Autodesk Inventor part; units mm, degrees
ref_plane "IDS_WORKPLANE{1}" through (-1.5513, 0, 0) normal (1, 0, 0) x (0, 0, -1)
ref_plane "Work Plane2" through (8.25, 0, 0) normal (0, 0, -1) x (1, 0, 0)
ref_plane "YZ Plane" through (0, 0, 0) normal (1, 0, 0) x (0, 1, 0)
sketch "Sketch1" plane through (0, 0, 0) normal (0, 0, 1) x (1, 0, 0)
  line L0 (-1.5513, 0) -> (5, 0)
  line L1 (5, 0) -> (5, 1.15)
  line L2 (5, 1.15) -> (1, 1.15)
  line L3 (1, 1.15) -> (0.7546, 1.0272)
  line L4 (0.7546, 1.0272) -> (0, 1.0272)
  line L5 (0, 1.0272) -> (0, 2)
  line L6 (-5.4046, 0) -> (21.3851, 0)
  line L7 (0, -0.4002) -> (0, 2.4013)
  line L8 (0, 2) -> (-1.4463, 1.9997)
  arc A0 (-1.4463, 1.9997) -> (-1.5513, 0) centre (17.558, 0) ccw
  dimension "d0" = 5
  dimension "d1" = 4
  dimension "d2" = 0.2454
  dimension "d3" = 1.5513
  dimension "d4" = 2.3
  dimension "d5" = 2.0545
  dimension "d9" = 4
  dimension "d10" = 0.01
  dimension "d15" = 19.1093
revolve "Body" add sketch "Sketch1" angle 360 about axis through (-1.5513, 0, 0) along (1, 0, 0)
fillet "Fillet1" radius 1.3 1 edges at (-1.4463, -1.9997, 0)
ref_plane "IDS_WORKPLANE{1}" through (-1.5513, 0, 0) normal (1, 0, 0) x (0, 0, -1)
sketch "Sketch2" plane through (-1.5513, 0, 0) normal (1, 0, 0) x (0, 0, -1)
  line L0 (0, -2.8) -> (0, 2.8)
  line L1 (2.8, 0) -> (-2.8, 0)
  line L2 (-2, 0.3) -> (2, 0.3)
  line L3 (2, 0.3) -> (2, -0.3)
  line L4 (2, -0.3) -> (-2, -0.3)
  line L5 (-2, -0.3) -> (-2, 0.3)
  line L6 (0, 0.3) -> (0, -0.3) construction
  line L7 (-2, 0) -> (2, 0) construction
  circle A0 centre (0, 0) radius 2
  dimension "d17" = 0.6
extrude "Slot" cut sketch "Sketch2" along normal blind 0.9 contours L4 A0 L1 L0 | L0 L1 A0 L4 | L4 L5 A0 | A0 L3 L4 | L1 A0 L2 L0 | L0 L2 A0 L1 | L5 L2 A0 | A0 L2 L3
thread "Thread"
chamfer "Chamfer1" distance 0.2454 distance2 0.2455 1 edges at (5, -1.15, 0) measured on face at (5, 0.3197, -0.0157)
ref_plane "Work Plane2" through (8.25, 0, 0) normal (0, 0, -1) x (1, 0, 0)
equation "\"d0\" = NLG"
equation "\"d1\" = GEL"
equation "\"d2\" = GAL"
equation "\"d3\" = KOH"
equation "\"d4\" = GD"
equation "\"d5\" = BDM"
equation "\"d9\" = KOD"
equation "\"d10\" = KEWI"
equation "\"d17\" = SBR"
equation "\"d18\" = STI"
equation "\"d20\" = RR"
equation "\"d11\" = GEL"
equation "\"d13\" = -0.5 * SPD + 0.5 * GD"
equation "\"GD\" = NND"
equation "\"NLG\" = 5"
equation "\"GEL\" = 4"
equation "\"KOD\" = 4"
equation "\"KOH\" = 1.55125"
equation "\"GAL\" = 0.61345 * PTC"
equation "\"SPD\" = NND - 1.2269 * PTC"
equation "\"BDM\" = 2.0545"
equation "\"GUL\" = 0.61345 * PTC"
equation "\"RR\" = 1.3"
equation "\"SBR\" = 0.6"
equation "\"STI\" = 0.9"
equation "\"KEWI\" = 0.01deg"
equation "\"KR\" = 2.4"
equation "\"d16\" = -KOH"
equation "\"PTC\" = 0.4"
equation "\"THREADDIA\" = 2.3"
equation "\"TOA\" = 30deg"
equation "\"NND\" = 2.3"
equation "\"ORI\" = 1.3"
equation "\"GD1\" = THREADDIA - 1.2269 * PTC"
properties part number "CNS 9671 - M2.3 x 5" material "Steel, Mild"
Check sheet for the modelled part. Datum: model origin and axes. Units: mm. A direction names the side the tool comes from. Round coordinates to 2 decimals unless told otherwise and drop trailing zeros. Write each loop counter-clockwise with the first axis right and the second up, starting at its lowest first coordinate (ties: lowest second). Pieces come first, ordered by that corner, then holes. Notation, with made-up numbers: M 79,-34 L 124,-34 A19 ccw 124,-11 Z; hole C -16,-29 d10. An arc over 180 degrees is marked long. Write item = value, one per line. Start each with the question number.
1. Gauge pin test, flat ends, axial feed: pin 1 (1.5 mm diameter, centred on x = 1.5, y = -0.5, fed in from +Z); pin 2 (0.7 mm diameter, centred on x = -1.5, z = 1, fed in from +Y); pin 3 (1 mm diameter, centred on x = -1, z = 0.5, fed in from -Y). Record the tip position at first contact, or that the pin passes through.
2. Section check A-A, the plane x = 4.5. Record the cut outline in (y, z).
3. Scan lines: line 1 (Y direction, x = 0.5, z = 0.05); line 2 (X direction, y = -0.4, z = 0.6); line 3 (Z direction, x = 4.5, y = -0.1). Record each from-to range of solid material in increasing order. Write a range as [from, to].
4. Tool access check on faces 1 (the cylindrical face through (2.85, -0.91, 0.7)), 2 (the flat face through (5, 0, 0)), 3 (the flat face through (-1, 0.3, 0)). Record the directions out of +Z, -Z, +X, -X, +Y, -Y that give a thin tool (end or side, any length) a straight path to the whole face; none if there is none.
5. Release check for a two-part mould opening along Y. For faces 4 (the cylindrical face through (0.37, 0.98, -0.31)), 5 (the flat face through (0, 1, -1)), 6 (the flat face through (-1, -0.3, 0)) record: pulls with the +Y half, pulls with the -Y half, needs draft (parallel to the pull), parting line crosses it, or undercut.
Results found:
q1.pin_1 = 1.15
q1.pin_2 = 1.35
q1.pin_3 = -1.94
q2.outline = C 0,0 d2.3
q3.line_1 = [-1.03, 1.03]
q3.line_2 = [-1.54, 5]
q3.line_3 = [-1.15, 1.15]
q4.face_1 = +X
q4.face_2 = +Z, -Z, +X, +Y, -Y
q4.face_3 = +Z, -Z, -X
q5.face_4 = parting line crosses it
q5.face_5 = needs draft
q5.face_6 = undercut
